from build123d import *

# Parameters (mm, degrees)
F0_W        = 206.1404287815
F0_H        = 88.9
F1_DEPTH    = 25.4
F4_D        = 50.8
F4_ON_F3_D  = 50.8
F5_W        = 88.9
F5_H        = 68.58
F6_DEPTH    = 25.401
F7_T        = 6.35
F7_T3_DEPTH = 38.1
F9_D        = 5.08
F9_DEPTH    = 3.175
F9_TIP      = 1.5261859723


# Not quite as in the source:
# - a shell that OpenCascade refuses in one call is made with other operations: the cavity is built on its own and cut out


with BuildPart() as f1:
    # F0 (on Front) → F1 (new body)
    with BuildSketch(Plane.XZ):
        Rectangle(F0_W, F0_H)
    extrude(amount=F1_DEPTH)

    # F4 (through all)
    with Locations(Plane.XZ.offset(25.4)):
        with Locations((-75.905919075, 0)):
            Hole(F4_D / 2)

    # F4 on F3 (through all)
    with Locations(Plane.XZ.offset(25.4)):
        with Locations((74.8937055469, 0)):
            Hole(F4_ON_F3_D / 2)

    # F5 (on face) → F6 (cut, through all)
    with BuildSketch(Plane.XZ.offset(25.4)):
        with Locations((-0.7901638031, 10.16)):
            Rectangle(F5_W, F5_H)
    extrude(amount=-F6_DEPTH, mode=Mode.SUBTRACT)

    # F7: shell of thickness 6.35, made by hand


with BuildPart() as f7_core1:
    # F7_t2: copy of F1
    add(f1.part)

    # the walls: a layer under each face that stays
    f7_faces = [f7_core1.faces().sort_by_distance(p)[0] for p in [
        (0, -12.7, -44.45),
        (-103.0702143908, -12.7, 0),
        (103.0702143908, -12.7, 0),
        (-68.7134762605, -25.4, -29.6333333333),
        (-74.1551890969, -12.7, 44.45),
        (73.3650252938, -12.7, 44.45),
        (-45.2401638031, -12.7, 10.16),
        (-0.7901638031, -12.7, -24.13),
        (43.6598361969, -12.7, 10.16),
        (-101.305919075, -12.7, 0),
        (49.4937055469, -12.7, 0),
    ]]
    thicken(f7_faces, amount=-F7_T, mode=Mode.SUBTRACT)

    # F7_s4 → F7_t3 (cut)
    with BuildSketch(Plane.XZ.offset(-6.35)):
        Polygon((-45.1766638031, -24.0665), (-51.5901638031, -24.13), (-51.5901638031, -30.48), (-45.2401638031, -30.48), align=None)
        Polygon((43.5963361969, -24.0665), (43.6598361969, -30.48), (50.0098361969, -30.48), (50.0098361969, -24.13), align=None)
    extrude(amount=F7_T3_DEPTH, mode=Mode.SUBTRACT)


with BuildPart() as f1_1:
    add(f1.part)

    # what is left inside the walls is the cavity
    f7_cavity = [f7_core1.part.solids().sort_by_distance(p)[0] for p in [
        (0, -12.7, -38.0365),
        (-73.404336, -6.35, 31.714994),
        (72.62573, -6.35, 31.732555),
    ]]
    add(f7_cavity, mode=Mode.SUBTRACT)

    # F9
    with Locations(Plane.XY.offset(-24.13)):
        with Locations((40.6420230865, -9.2453807592), (33.507373184, -9.2453807592), (26.3727232814, -9.2453807592), (19.2380733788, -9.2453807592), (12.8678502515, -9.2453807592)):
            Hole(F9_D / 2, depth=F9_DEPTH)
            with Locations((0, 0, -(F9_DEPTH + F9_TIP / 2))):  # 118° drill point
                Cone(0, F9_D / 2, F9_TIP, mode=Mode.SUBTRACT)


solid = f1_1.part
Read the model definition and answer for the solid it produces. Units are mm, in the model's axes. A direction names the side the tool comes from. Coordinates: 2 decimals unless noted, no trailing zeros. Order: outer loops, then holes, each group sorted by start corner. A loop starts at its lowest first (then second) coordinate and runs counter-clockwise, first axis right, second up. Notation, with made-up numbers: M -1.75,-16 L 38.25,-16 A10 ccw 38.25,-9 Z; hole C 19.5,23.5 d4. An arc over 180 degrees is marked long. Put each result on its own line as item: value. Start each with the question number.
Item 1: For faces 5 (the face through (-50.53, -12.52, 1.12)), 6 (the face through (-1, -9, -38.1)), 7 (the face through (36.045, -9.134, -25.74)), determine the directions among +Z, -Z, +X, -X, +Y, -Y from which every point of the face is accessible in a straight line to the end or side of a thin tool.
Item 2: Section C-C, the plane x = 54 is taken. Determine the outline of the cut face in (y, z), plus the area to 3 significant figures.
Item 3: Section A-A, the plane y = -23 is taken. Determine the outline of the cut face in (x, z), plus the area to 3 significant figures.
Item 4: Section D-D, the plane y = -2.25 is taken. Determine the outline of the cut face in (x, z).
Item 5: Section B-B, the plane z = 0 is taken. Determine the outline of the cut face in (x, y), plus the area to 3 significant figures.
Item 6: Consider probe 1 along Z at (x, y) = (73.5, -5); probe 2 along Z at (x, y) = (-32, -13); probe 3 along X at (y, z) = (-15.75, 4). Determine where each line is inside the solid, lowest interval first. Write a range as [from, to].
Item 7: Given pin 1 Ø4 at (x, y) = (19.24, -9.25) entering from +Z; pin 2 Ø6 at (x, y) = (26.37, -9.25) entering from +Z, each flat-ended and moving along its own axis, determine where each tip first touches the part or whether it passes through.
Item 8: The mould has two halves that part along X. Classify faces 1 (the face through (-96.72, -9, 31)), 2 (the face through (103.07, -13, -1)), 3 (the face through (73, -19.05, 33)), 4 (the face through (-1, -25.4, -29)): +X half, -X half, draft (parallel to the pull), parting line (faces both ways), or undercut.
Computed:
1. face 5: +Y, -Y
1. face 6: +Y
1. face 7: +Z
2. outline: M -25.4,-44.45 L 0,-44.45 L 0,-38.1 L -19.05,-38.1 L -19.05,-23.91 L 0,-23.91 L 0,-14.44 L -25.4,-14.44 Z; M -25.4,14.44 L 0,14.44 L 0,23.91 L -19.05,23.91 L -19.05,38.1 L 0,38.1 L 0,44.45 L -25.4,44.45 Z
2. area: 984 mm2
3. outline: M -103.07,-44.45 L 103.07,-44.45 L 103.07,44.45 L 43.66,44.45 L 43.66,-24.13 L -45.24,-24.13 L -45.24,44.45 L -103.07,44.45 Z; hole C -75.91,0 d50.8; hole C 74.89,0 d50.8
3. area: 8,180 mm2
4. outline: M -103.07,-44.45 L 103.07,-44.45 L 103.07,44.45 L 43.66,44.45 L 43.66,-24.13 L -45.24,-24.13 L -45.24,44.45 L -103.07,44.45 Z; hole C -75.91,0 d50.8; hole M -96.72,-38.1 L 96.72,-38.1 L 96.72,-23.06 A31.75 cw 50.01,-19.72 L 50.01,-30.48 L -51.59,-30.48 L -51.59,-20.42 A31.75 cw -96.72,-23.98 Z; hole M -96.72,23.98 A31.75 cw -51.59,20.42 L -51.59,38.1 L -96.72,38.1 Z; hole C 74.89,0 d50.8; hole M 50.01,19.72 A31.75 cw 96.72,23.06 L 96.72,38.1 L 50.01,38.1 Z
5. outline: M -103.07,-25.4 L -101.31,-25.4 L -101.31,0 L -103.07,0 Z; M -50.51,-25.4 L -45.24,-25.4 L -45.24,0 L -50.51,0 Z; M 43.66,-25.4 L 49.49,-25.4 L 49.49,0 L 43.66,0 Z; M 100.29,-25.4 L 103.07,-25.4 L 103.07,0 L 100.29,0 Z
5. area: 397 mm2
6. probe 1: z = [-44.45, -38.1], [-31.72, -25.36], [25.36, 31.72], [38.1, 44.45]
6. probe 2: z = [-44.45, -38.1], [-30.48, -24.13]
6. probe 3: x = [-103.07, -100.99], [-50.82, -45.24], [43.66, 49.81], [99.98, 103.07]
7. pin 1: stops at z = -27.63
7. pin 2: stops at z = -24.13
8. face 1: undercut
8. face 2: +X half
8. face 3: undercut
8. face 4: draft
